Input: dimensioned drawing with shaded views. Units: mm. Origin: part minimum x, y, z. Round coordinates to 2 decimals unless told otherwise and drop trailing zeros. Loops run counter-clockwise (first coordinate to the right, second up) from the corner with the lowest first, then second, coordinate; pieces in that order, holes last.
1) Section C-C, the plane x = 60. Return loops of the section in (y, z).
2) Section B-B, the plane y = 160.5. Return loops of the section in (x, z).
3) Ray query, line 1 along X through (y, z) = (166, 4); line 2 along X through (y, z) = (56.5, 4); line 3 along Y through (x, z) = (63.5, 4.5) (1 decimal). Return the intervals inside material, ascending.
4) First-contact query: pin 1 (1 mm diameter, centred on x = 34, z = 3.5, fed in from -Y); pin 2 (4 mm diameter, centred on y = 156, z = 5.5, fed in from -X); pin 3 (2.5 mm diameter, centred on y = 153, z = 4, fed in from +X). Flat tips, straight axial feed; report the tip coordinate or a pass-through.
5) Section A-A, the plane z = 4.5. Return loops of the section in (x, y).
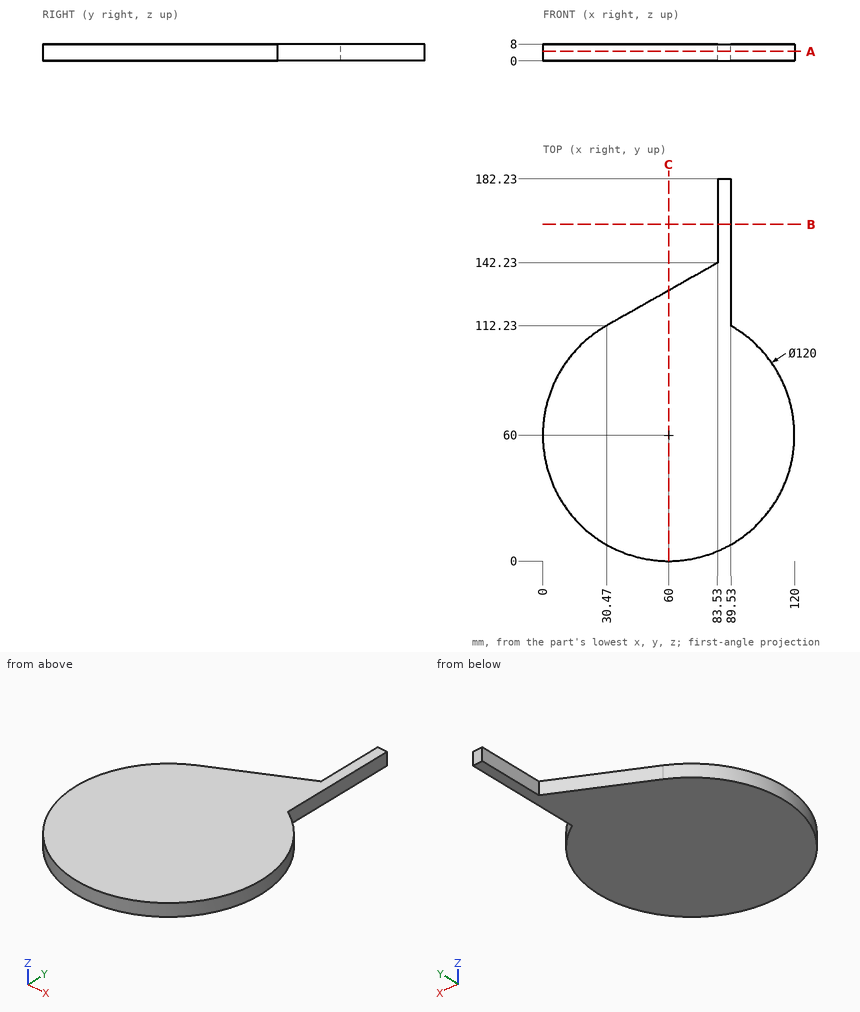
Final values:
1. outline: (0, 0) - (128.93, 0) - (128.93, 8) - (0, 8) - close
2. outline: (83.53, 0) - (89.53, 0) - (89.53, 8) - (83.53, 8) - close
3. line 1: x = 83.53 to 89.53
3. line 2: x = 0.1 to 119.9
3. line 3: y = 0.1 to 130.9
4. pin 1: stops at y = 5.69
4. pin 2: stops at x = 83.53
4. pin 3: stops at x = 89.53
5. outline: (30.47, 112.23) arc R60 ccw (long way) to (89.53, 112.23) - (89.53, 182.23) - (83.53, 182.23) - (83.53, 142.23) - close
